Can you work these out from the model? Positions are in its coordinate system, mm. Face numbers are marked on the shaded views. A direction names the side the tool comes from. Give positions to 0.01 mm unless a question says otherwise; leave off trailing zeros. Order: outer loops, then holes, each group sorted by start corner. A loop starts at its lowest first (then second) coordinate and runs counter-clockwise, first axis right, second up.
Item 1: If we mould it in two halves opening along X, with no side actions, what happens to the marked faces 1, 2 and 3? For each: +X half, -X half, draft (parallel to the pull), parting line (faces both ways), or undercut.
Item 2: If I drill on line 1 along X through (y, z) = (2.5, -0.75); line 2 along X through (y, z) = (-2, -2); line 3 along Y through (x, z) = (1.55, -0.25), over which ranges is the centre line in solid material (lowest first)?
Item 3: I want a section at B-B, the plane z = 4. Write out the boundary of the cut face in (x, y), then the cut area to 3 significant figures.
Item 4: I want a section at D-D, the plane y = -2.5. Write out the boundary of the cut face in (x, z), then the cut area to 3 significant figures.
Item 5: Which directions (+Z, -Z, +X, -X, +Y, -Y) give clear straight access to the entire face, cutting with the end or side of a thin tool? Please do the marked faces 4, 5 and 6.
Item 6: I'm going to push flat-ended pins straight in: pin 1 Ø2 at (x, z) = (2, -2.5) entering from -Y; pin 2 Ø1.6 at (y, z) = (-1, 0.5) entering from -X; pin 3 Ø0.9 at (y, z) = (-1, 0.5) entering from +X. Where does each tip first touch, or does it pass through?
Item 7: I want a section at A-A, the plane y = 1. Write out the boundary of the cut face in (x, z), then the cut area to 3 significant figures.
Item 8: I want a section at C-C, the plane x = -1.15. Write out the boundary of the cut face in (y, z), then the cut area to 3 significant figures.
Autodesk Inventor part; units mm, degrees
ref_plane "YZ Plane" through (0, 0, 0) normal (1, 0, 0) x (0, 1, 0)
ref_plane "XZ Plane" through (0, 0, 0) normal (0, 1, 0) x (-1, 0, 0)
ref_plane "XY Plane" through (0, 0, 0) normal (0, 0, 1) x (1, 0, 0)
sketch "스케치1" plane through (0, 0, 0) normal (0, 1, 0) x (-1, 0, 0)
  line L0 (-2.4, 4.8) -> (2.4, 4.8)
  line L1 (2.4, 4.8) -> (2.4, -4.8)
  line L2 (2.4, -4.8) -> (-2.4, -4.8)
  line L3 (-2.4, -4.8) -> (-2.4, 4.8)
  line L4 (-2.4, 4.8) -> (2.4, -4.8) construction
  line L5 (2.4, 4.8) -> (-2.4, -4.8) construction
  point P0 (0, 0)
  dimension "d0" = 4.8
  dimension "d1" = 9.6
extrude "돌출1" add sketch "스케치1" along normal blind 0.6
sketch "스케치2" plane through (0, 0, 0) normal (0, -1, 0) x (1, 0, 0)
  line L0 (2.4, -4.8) -> (-2.4, -4.8)
  line L1 (2.4, 4.8) -> (2.4, -4.8)
  line L2 (-2.4, 4.8) -> (2.4, 4.8)
  line L3 (-2.4, -4.8) -> (-2.4, 4.8)
  line L4 (2.4, 4.8) -> (3, 4.8)
  line L5 (3, 4.8) -> (3, -4.8)
  line L6 (3, -4.8) -> (2.4, -4.8)
  line L7 (2.4, -4.8) -> (2.4, 4.8)
  line L8 (-2.4, -4.8) -> (-2.4, 4.8)
  line L9 (-2.4, 4.8) -> (-3, 4.8)
  line L10 (-3, 4.8) -> (-3, -4.8)
  line L11 (-3, -4.8) -> (-2.4, -4.8)
  line L12 (-2.4, -4.8) -> (-2.4, 4.8)
  point P0 (0, 0)
  dimension "d4" = 0.6
  dimension "d5" = 0.6
extrude "돌출2" add sketch "스케치2" against normal blind 3.1 contours L1 L4 L5 L6 | L11 L10 L9 L3
sketch "스케치3" plane through (0, 0, 0) normal (0, -1, 0) x (1, 0, 0)
  line L0 (2.4, -4.8) -> (-2.4, -4.8)
  line L1 (-0.5, 4.8) -> (0.5, 4.8)
  line L2 (0.5, 4.8) -> (0.5, -4.8)
  line L3 (0.5, -4.8) -> (-0.5, -4.8)
  line L4 (-0.5, -4.8) -> (-0.5, 4.8)
  line L5 (-0.5, 4.8) -> (0.5, -4.8) construction
  line L6 (0.5, 4.8) -> (-0.5, -4.8) construction
  point P0 (0, 0)
  dimension "d8" = 1
extrude "돌출3" add sketch "스케치3" along normal blind 3.1
chamfer "모따기1" distance 1 angle 45 2 edges at (-0.5, 0, 0) (0.5, 0, 0)
sketch "스케치4" plane through (0, -3.1, 0) normal (0, -1, 0) x (1, 0, 0)
  line L0 (1.5, 4.8) -> (0.5, 4.8)
  line L1 (0.5, 4.8) -> (0.5, -4.8)
  line L2 (0.5, -4.8) -> (1.5, -4.8)
  line L3 (1.5, -4.8) -> (1.5, 4.8)
  line L4 (-0.5, 4.8) -> (-0.5, -4.8)
  line L5 (-0.5, -4.8) -> (0.5, -4.8)
  line L6 (0.5, -4.8) -> (0.5, 4.8)
  line L7 (0.5, 4.8) -> (-0.5, 4.8)
  line L8 (-1.5, -4.8) -> (-0.5, -4.8)
  line L9 (-0.5, -4.8) -> (-0.5, 4.8)
  line L10 (-0.5, 4.8) -> (-1.5, 4.8)
  line L11 (-1.5, 4.8) -> (-1.5, -4.8)
  line L12 (-1.5, 1.6) -> (1.5, 1.6)
  line L13 (1.5, 1.6) -> (1.5, -1.6)
  line L14 (1.5, -1.6) -> (-1.5, -1.6)
  line L15 (-1.5, -1.6) -> (-1.5, 1.6)
  line L16 (-1.5, 1.6) -> (1.5, -1.6) construction
  line L17 (1.5, 1.6) -> (-1.5, -1.6) construction
  point P0 (0, 0)
  point P1 (-0.5, -1.6)
  point P2 (-0.5, 1.6)
  point P3 (0.5, -1.6)
  point P4 (0.5, 1.6)
  dimension "d14" = 3.2
extrude "돌출4" cut sketch "스케치4" against normal up to surface (3.1 mm away) contours L3 L14 L1 L12 | L4 L14 L11 L12
properties part number "endcap_4mm_2ea_addon_large"
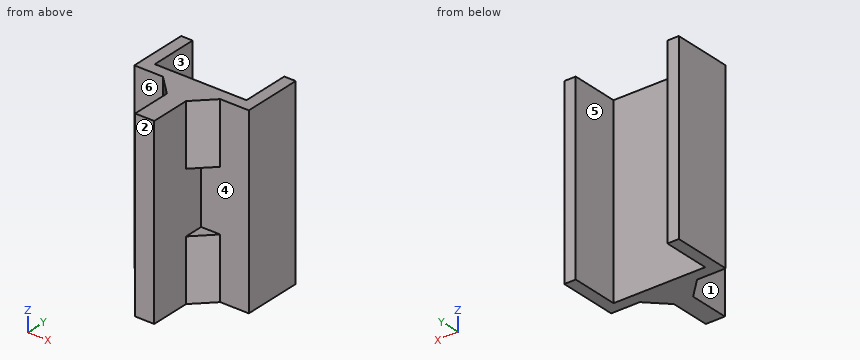
Results list:
1. face 1: -X half
1. face 2: draft
1. face 3: undercut
2. line 1: x = -3 to -2.4, 2.4 to 3
2. line 2: x = -0.5 to 0.5
2. line 3: y = 0 to 0.6
3. outline: (-3, 0) - (-1.5, 0) - (-0.5, -1) - (-0.5, -3.1) - (0.5, -3.1) - (0.5, -1) - (1.5, 0) - (3, 0) - (3, 3.1) - (2.4, 3.1) - (2.4, 0.6) - (-2.4, 0.6) - (-2.4, 3.1) - (-3, 3.1) - close
3. area: 10.7 mm2
4. outline: (-0.5, -4.8) - (0.5, -4.8) - (0.5, 4.8) - (-0.5, 4.8) - close
4. area: 9.60 mm2
5. face 4: +X, -Y
5. face 5: +Z, -Z, +Y
5. face 6: -X, -Y
6. pin 1: stops at y = -0.5
6. pin 2: stops at x = -0.5
6. pin 3: stops at x = 0.5
7. outline: (-3, -4.8) - (-2.4, -4.8) - (-2.4, 4.8) - (-3, 4.8) - close; (2.4, -4.8) - (3, -4.8) - (3, 4.8) - (2.4, 4.8) - close
7. area: 11.5 mm2
8. outline: (-0.35, -4.8) - (0.6, -4.8) - (0.6, 4.8) - (-0.35, 4.8) - (-0.35, 1.6) - (0, 1.6) - (0, -1.6) - (-0.35, -1.6) - close
8. area: 8.00 mm2
